Geometry check sheet. Reference: the model listing, model coordinates, mm. Face numbers are marked on the shaded views. A direction names the side the tool comes from. Give positions to 0.01 mm unless a question says otherwise; leave off trailing zeros. Loops run counter-clockwise (first coordinate to the right, second up) from the corner with the lowest first, then second, coordinate; pieces in that order, holes last. Notation, with made-up numbers: (11, 23) -> (20, 23) arc R17 cw to (20, 39) -> close; hole circle Ø2 at (57, 85). An arc over 180 degrees is marked (long way). Write each question's results on one line, items separated by ' | '. Start each with the question number.
1) Depth check by flat-ended pin: pin 1 (1.5 mm diameter, centred on x = -16.5, z = 16.5, fed in from +Y); pin 2 (3 mm diameter, centred on y = 22, z = -4.5, fed in from +X); pin 3 (1 mm diameter, centred on x = 0.5, z = 22.5, fed in from -Y). Enter the tip coordinate at first touch or a pass-through.
2) Sectioned sample at C-C on z = 0. Record the cut outline in (x, y), then the cut area to 3 significant figures.
3) Sectioned sample at D-D on z = -10. Record the cut outline in (x, y).
4) Sectioned sample at B-B on y = 29. Record the cut outline in (x, z).
5) Set-up check for the marked faces 1, 2, 3, 4 and 5: record each of +Z, -Z, +X, -X, +Y, -Y from which the full face is reachable in a straight line by a thin tool's end or side.
6) Draft check along Y on the marked faces 6, 7, 8 and 9. Enter one of: pulls with the +Y half, pulls with the -Y half, needs draft (parallel to the pull), parting line crosses it, or undercut.
7) Scan lines: line 1 (Z direction, x = -15.5, y = 39.9); line 2 (X direction, y = 3.4, z = 15.5). Record each from-to range of solid material in increasing order. Write a range as from..to.
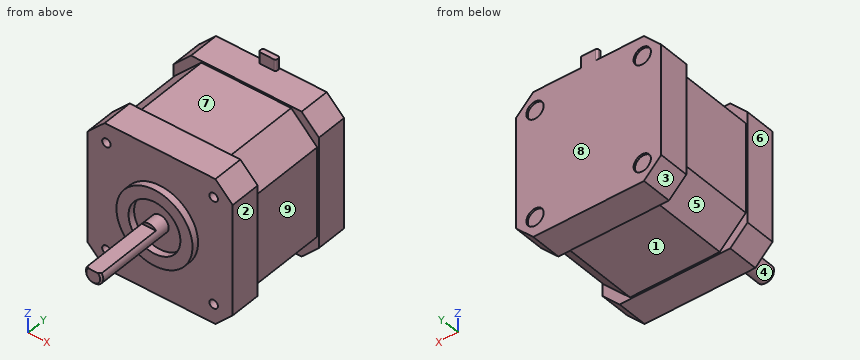
```python
from build123d import *

# Parameters (mm, degrees)
ESQUISSE1_W                         = 42
ESQUISSE1_H                         = 9
BOSS_EXTRU_1_DEPTH                  = 0.5
BOSS_EXTRU_2_DEPTH                  = 41
ESQUISSE3_W                         = 42
ESQUISSE3_H                         = 9
BOSS_EXTRU_3_DEPTH                  = 0.5
ESQUISSE4_W                         = 42
ESQUISSE4_H                         = 42
BOSS_EXTRU_4_DEPTH                  = 9
ESQUISSE5_W                         = 5
ESQUISSE5_H                         = 1.5
BOSS_EXTRU_5_DEPTH                  = 3.2869072
ESQUISSE6_R                         = 11
BOSS_EXTRU_6_DEPTH                  = 2
DIAM_TRE_DU_PER_AGE_15_0_15_1_D     = 15
DIAM_TRE_DU_PER_AGE_15_0_15_1_DEPTH = 2
ESQUISSE9_R                         = 2.5
BOSS_EXTRU_7_DEPTH                  = 24
ENL_V_START                         = -20
ENL_V_MAT_EXTRU_1_DEPTH             = 20
DIAM_TRE_DU_PER_AGE_5_0_5_1_D       = 5
DIAM_TRE_DU_PER_AGE_5_0_5_1_DEPTH   = 0.5
D_GAGEMENT_M21_D                    = 2.459
D_GAGEMENT_M21_DEPTH                = 4.5
CHANFREIN1_SIZE                     = 7.535533906
CHANFREIN2_SIZE                     = 5
CHANFREIN3_SIZE                     = 0.5
CONG_1_R                            = 0.5


with BuildPart() as part:
    # Esquisse1 → Boss.-Extru.1 (new body)
    with BuildSketch(Plane.XY.offset(21)):
        with Locations((0, 4.5)):
            Rectangle(ESQUISSE1_W, ESQUISSE1_H)
    extrude(amount=-BOSS_EXTRU_1_DEPTH)

    # Esquisse2 → Boss.-Extru.2 (add)
    with BuildSketch(Plane(origin=(0, 0, 20.5), x_dir=(-1, 0, 0), z_dir=(0, 0, -1))):
        Polygon((-20.5, 9), (-20.5, 31), (20.5, 31), (20.5, 9), (21, 9), (21, 0), (-21, 0), (-21, 9), align=None)
    extrude(amount=BOSS_EXTRU_2_DEPTH)

    # Esquisse3 → Boss.-Extru.3 (add)
    with BuildSketch(Plane(origin=(0, 0, -20.5), x_dir=(-1, 0, 0), z_dir=(0, 0, -1))):
        with Locations((0, 4.5)):
            Rectangle(ESQUISSE3_W, ESQUISSE3_H)
    extrude(amount=BOSS_EXTRU_3_DEPTH)

    # Esquisse4 → Boss.-Extru.4 (add)
    with BuildSketch(Plane.XZ.offset(-31)):
        Rectangle(ESQUISSE4_W, ESQUISSE4_H)
    extrude(amount=-BOSS_EXTRU_4_DEPTH)

    # Esquisse5 → Boss.-Extru.5 (add)
    with BuildSketch(Plane.XY.offset(21)):
        with Locations((0, 39.25)):
            Rectangle(ESQUISSE5_W, ESQUISSE5_H)
    extrude(amount=BOSS_EXTRU_5_DEPTH)

    # Esquisse6 → Boss.-Extru.6 (add)
    with BuildSketch(Plane.XZ):
        with Locations(Location((0, 0, 0), (0, 0, 270))):
            Circle(ESQUISSE6_R)
    extrude(amount=BOSS_EXTRU_6_DEPTH)

    # Diamètre du perçage Ø15.0 (15)1
    with Locations(Plane(origin=(0, -2, 0), x_dir=(-1, 0, 0), z_dir=(0, -1, 0))):
        with Locations((0, 0)):
            Hole(DIAM_TRE_DU_PER_AGE_15_0_15_1_D / 2, depth=DIAM_TRE_DU_PER_AGE_15_0_15_1_DEPTH)

    # Esquisse9 → Boss.-Extru.7 (add)
    with BuildSketch(Plane.XZ):
        with Locations(Location((0, 0, 0), (0, 0, 90))):
            Circle(ESQUISSE9_R)
    extrude(amount=BOSS_EXTRU_7_DEPTH)

    # Esquisse10 → Enlèv. mat.-Extru.1 (cut)
    with BuildSketch(Plane.XZ.offset(24).offset(ENL_V_START)):
        with BuildLine():
            Line((-2.038647634, 1.447036912), (2.038647634, 1.447036912))
            ThreePointArc((2.038647634, 1.447036912), (0, 2.5), (-2.038647634, 1.447036912))
        make_face()
    extrude(amount=ENL_V_MAT_EXTRU_1_DEPTH, mode=Mode.SUBTRACT)

    # Diamètre du perçage Ø5.0 (5)1
    with Locations(Plane(origin=(0, 40, 0), x_dir=(1, 0, 0), z_dir=(0, 1, 0))):
        with Locations((15.5, -15.5), (-15.5, -15.5), (-15.5, 15.5), (15.5, 15.5)):
            Hole(DIAM_TRE_DU_PER_AGE_5_0_5_1_D / 2, depth=DIAM_TRE_DU_PER_AGE_5_0_5_1_DEPTH)

    # Dégagement M21
    with Locations(Plane(origin=(0, 0, 0), x_dir=(-1, 0, 0), z_dir=(0, -1, 0))):
        with Locations((15.5, -15.5), (-15.5, -15.5), (-15.5, 15.5), (15.5, 15.5)):
            Hole(D_GAGEMENT_M21_D / 2, depth=D_GAGEMENT_M21_DEPTH)

    # Chanfrein1
    chanfrein1_edges = [part.edges().sort_by_distance(p)[0] for p in [
        (-20.5, 20, 20.5),
        (20.5, 20, 20.5),
        (-20.5, 20, -20.5),
        (20.5, 20, -20.5),
    ]]
    chamfer(chanfrein1_edges, length=CHANFREIN1_SIZE)

    # Chanfrein2
    chanfrein2_edges = [part.edges().sort_by_distance(p)[0] for p in [
        (21, 4.5, -21),
        (-21, 4.5, -21),
        (-21, 35.5, 21),
        (21, 35.5, 21),
        (21, 35.5, -21),
        (-21, 35.5, -21),
        (-21, 4.5, 21),
        (21, 4.5, 21),
    ]]
    chamfer(chanfrein2_edges, length=CHANFREIN2_SIZE)

    # Chanfrein3
    chanfrein3_edges = [part.edges().sort_by_distance(p)[0] for p in [
        (0, -24, -2.5),
    ]]
    chamfer(chanfrein3_edges, length=CHANFREIN3_SIZE)

    # Congé1
    cong_1_edges = [part.edges().sort_by_distance(p)[0] for p in [
        (-2.5, 40, 22.6434536),
        (-2.5, 38.5, 22.6434536),
        (2.5, 38.5, 22.6434536),
        (2.5, 40, 22.6434536),
    ]]
    fillet(cong_1_edges, radius=CONG_1_R)


solid = part.part
```
Result:
1) pin 1: y = 39.5 | pin 2: x = 20.5 | pin 3: y = 38.5
2) outline: (-21, 0) -> (-11, 0) -> (-11, -2) -> (-7.5, -2) -> (-7.5, 0) -> (-2.5, 0) -> (-2.5, -23.5) -> (-2, -24) -> (2, -24) -> (2.5, -23.5) -> (2.5, 0) -> (7.5, 0) -> (7.5, -2) -> (11, -2) -> (11, 0) -> (21, 0) -> (21, 9) -> (20.5, 9) -> (20.5, 31) -> (21, 31) -> (21, 40) -> (-21, 40) -> (-21, 31) -> (-20.5, 31) -> (-20.5, 9) -> (-21, 9) -> close | area: 1,790 mm^2
3) outline: (-21, 0) -> (-4.58, 0) -> (-4.58, -2) -> (4.58, -2) -> (4.58, 0) -> (21, 0) -> (21, 9) -> (20.5, 9) -> (20.5, 31) -> (21, 31) -> (21, 40) -> (-21, 40) -> (-21, 31) -> (-20.5, 31) -> (-20.5, 9) -> (-21, 9) -> close
4) outline: (-20.5, -12.96) -> (-12.96, -20.5) -> (12.96, -20.5) -> (20.5, -12.96) -> (20.5, 12.96) -> (12.96, 20.5) -> (-12.96, 20.5) -> (-20.5, 12.96) -> close
5) face 1: -Z, +X, -X | face 2: +Z, -Z, +X, +Y, -Y | face 3: -Z, -X, +Y, -Y | face 4: -Y | face 5: -Z, -X
6) face 6: needs draft | face 7: undercut | face 8: pulls with the +Y half | face 9: undercut
7) line 1: -21..-18, -13..13, 18..21 | line 2: -21..-16.73, -14.27..14.27, 16.73..21
